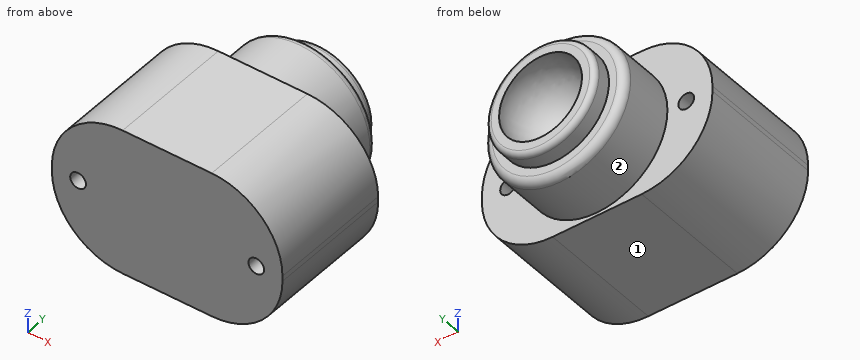
```python
from build123d import *

# Parameters (mm, degrees)
FILLET1_R           = 1
FILLET2_R           = 1.5
SKETCH5_W           = 44
SKETCH5_H           = 28
BOSS_EXTRUDE1_DEPTH = 24
FILLET3_R           = 13.5
SKETCH7_R           = 1.5
CUT_EXTRUDE1_DEPTH  = 25


with BuildPart() as part:
    # Sketch1 → Revolve2 (revolve)
    with BuildSketch(Plane.XY):
        with BuildLine():
            Line((0, 0), (0, 5))
            ThreePointArc((0, 5), (6.071429533, 7.79069576), (7.907014302, 14.215714666))
            Line((7.907014302, 14.215714666), (10.407014302, 14.215714666))
            Line((10.407014302, 14.215714666), (10.407014302, 10.715714666))
            Line((10.407014302, 10.715714666), (13.407014302, 10.715714666))
            Line((13.407014302, 10.715714666), (13.407014302, 0))
            Line((13.407014302, 0), (0, 0))
        make_face()
    revolve(axis=Axis((0, 0, 0), (0, 1, 0)))

    # Fillet1
    fillet1_edges = [part.edges().sort_by_distance(p)[0] for p in [
        (-10.407014302, 14.215714666, 0),
    ]]
    fillet(fillet1_edges, radius=FILLET1_R)

    # Fillet2
    fillet2_edges = [part.edges().sort_by_distance(p)[0] for p in [
        (-13.407014302, 10.715714666, 0),
    ]]
    fillet(fillet2_edges, radius=FILLET2_R)

    # Sketch5 → Boss-Extrude1 (add)
    with BuildSketch(Plane(origin=(0, 0, 0), x_dir=(1, 0, 0), z_dir=(0, 1, 0))):
        Rectangle(SKETCH5_W, SKETCH5_H)
    extrude(amount=-BOSS_EXTRUDE1_DEPTH)

    # Fillet3
    fillet3_edges = [part.edges().sort_by_distance(p)[0] for p in [
        (-22, -12, 14),
        (-22, -12, -14),
        (22, -12, -14),
        (22, -12, 14),
    ]]
    fillet(fillet3_edges, radius=FILLET3_R)

    # Sketch7 → Cut-Extrude1 (cut, through all)
    with BuildSketch(Plane(origin=(0, 0, 0), x_dir=(1, 0, 0), z_dir=(0, 1, 0))):
        with Locations((-17, 0)):
            Circle(SKETCH7_R)
    cut_extrude1 = extrude(amount=-CUT_EXTRUDE1_DEPTH, mode=Mode.SUBTRACT)

    # Mirror1: Cut-Extrude1 across plane
    add(cut_extrude1.mirror(Plane.ZY), mode=Mode.SUBTRACT)


solid = part.part
```
Design review of the part built by this model. Coordinates are the model's own, in mm. Face numbers are marked on the shaded views. A direction names the side the tool comes from. Give positions to 0.01 mm unless a question says otherwise; leave off trailing zeros. Order: outer loops, then holes, each group sorted by start corner. A loop starts at its lowest first (then second) coordinate and runs counter-clockwise, first axis right, second up. Notation, with made-up numbers: (-26, 47.25) -> (-9, 47.25) arc R16 ccw to (-9, 52.25) -> close; hole circle Ø10 at (-36.5, 23.25). An arc over 180 degrees is marked (long way). Write item = value, one per line. Start each with the question number.
(1) For the marked faces 1 and 2, list the 3-axis set-ups (+Z, -Z, +X, -X, +Y, -Y) from which the entire face can be reached by the end or side of a thin tool; tool diameter is ignored.
(2) For pin 1 (6 mm diameter, centred on y = -5, z = -10.5, fed in from +X); pin 2 (3 mm diameter, centred on x = -12.5, y = 8.5, fed in from -Z); pin 3 (2.5 mm diameter, centred on x = -17, z = 0, fed in from -Y); pin 4 (4 mm diameter, centred on x = 17, z = 0, fed in from +Y), all flat-tipped, find the tip position at first contact; note any pin that passes through.
(3) We need section B-B on x = 17. Write out the cut boundary in (y, z), plus the area to 3 significant figures.
(4) To check wall thickness, follow line 1 along X through (y, z) = (-12, 0); line 2 along X through (y, z) = (-19, -0.5); line 3 along Y through (x, z) = (-11.5, -7.75). State the ranges of each line that lie inside material, in increasing order.
(5) We need section C-C on y = 2.5. Write out the cut boundary in (x, z).
(6) We need section A-A on y = -16. Write out the cut boundary in (x, z).
(7) We need section D-D on x = -14. Write out the cut boundary in (y, z).
Numbers:
q1.face_1 = -Z, +X, -X, +Y, -Y
q1.face_2 = +Y
q2.pin_1 = 20.04
q2.pin_2 = -7.66
q2.pin_3 = through
q2.pin_4 = 0
q3.outline = (-24, -10.99) -> (0, -10.99) -> (0, -1.5) -> (-24, -1.5) -> close; (-24, 1.5) -> (0, 1.5) -> (0, 10.99) -> (-24, 10.99) -> close
q3.area = 455 mm^2
q4.line_1 = -22 to -18.5, -15.5 to 15.5, 18.5 to 22
q4.line_2 = -22 to -18.41, -15.59 to 15.59, 18.41 to 22
q4.line_3 = -24 to 0
q5.outline = circle Ø26.81 at (0, 0)
q6.outline = (-22, -0.5) arc R13.5 ccw to (-8.5, -14) -> (8.5, -14) arc R13.5 ccw to (22, -0.5) -> (22, 0.5) arc R13.5 ccw to (8.5, 14) -> (-8.5, 14) arc R13.5 ccw to (-22, 0.5) -> close; hole circle Ø3 at (-17, 0); hole circle Ø3 at (17, 0)
q7.outline = (-24, -12.83) -> (0, -12.83) -> (0, 12.83) -> (-24, 12.83) -> close
